Design review of the part built by this model. Coordinates are the model's own, in mm. A direction names the side the tool comes from. Give positions to 0.01 mm unless a question says otherwise; leave off trailing zeros. Write each loop counter-clockwise with the first axis right and the second up, starting at its lowest first coordinate (ties: lowest second). Pieces come first, ordered by that corner, then holes. Notation, with made-up numbers: (53.5, -13.75) -> (76.5, -13.75) arc R22 ccw to (76.5, 19.25) -> close; hole circle Ø4 at (68.25, 47). An arc over 180 degrees is marked (long way). Answer as a JSON object with one key per item and string values.
Autodesk Inventor part; units mm, degrees
ref_plane "YZ Plane" through (0, 0, 0) normal (1, 0, 0) x (0, 1, 0)
ref_plane "XZ Plane" through (0, 0, 0) normal (0, 1, 0) x (-1, 0, 0)
ref_plane "XY Plane" through (0, 0, 0) normal (0, 0, 1) x (1, 0, 0)
sketch "스케치1" plane through (0, 0, 0) normal (1, 0, 0) x (0, 1, 0)
  line L0 (0, 0) -> (15, 0)
  line L1 (15, 0) -> (15, -11)
  line L2 (15, -11) -> (0, -11)
  line L3 (0, -11) -> (0, 0)
  line L4 (15, -11) -> (8.9773, -11)
  line L5 (10, -9.9773) -> (15, -9.9773)
  line L6 (15, -9.9773) -> (15, -11)
  line L7 (0, -11) -> (5, -11)
  line L8 (0, -10) -> (0, -11)
  line L9 (5, -11) -> (7, -11)
  line L10 (7, -11) -> (8, -11)
  line L11 (8, -11) -> (8, -10.5)
  line L12 (8.9773, -11) -> (10, -9.9773)
  line L13 (8.9773, -11) -> (10.4236, -11) construction
  line L14 (7, -11) -> (7.5, -10.5)
  line L15 (8, -10.5) -> (7.5, -10.5)
  dimension "d0" = 15
  dimension "d1" = 11
  dimension "d8" = 45
  dimension "d9" = 5
extrude "돌출1" add sketch "스케치1" along normal blind 1 contours L0 L1 L5 L12 L2 L11 L15 L14 L3
fillet "모깎기1" radius 1 4 edges at (0.5, 15, -9.9773) (0.5, 15, 0) (0.5, 0, -11) (0.5, 0, 0)
sketch "스케치2" plane through (1, 0, 0) normal (1, 0, 0) x (0, 0, -1)
  arc A0 (0, 1) -> (1, 0) centre (1, 1) ccw
  line L0 (1, 0) -> (10, 0)
  arc A1 (10, 0) -> (11, 1) centre (10, 1) ccw
  line L1 (11, 1) -> (11, 7)
  line L2 (11, 7) -> (10.5, 7.5)
  line L3 (10.5, 7.5) -> (10.5, 8)
  line L4 (10.5, 8) -> (11, 8)
  line L5 (11, 8) -> (11, 8.9773)
  line L6 (11, 8.9773) -> (9.9773, 10)
  line L7 (9.9773, 10) -> (9.9773, 14)
  arc A2 (9.9773, 14) -> (8.9773, 15) centre (8.9773, 14) ccw
  line L8 (8.9773, 15) -> (1, 15)
  arc A3 (1, 15) -> (0, 14) centre (1, 14) ccw
  line L9 (0, 14) -> (0, 1)
  line L10 (-0.1139, -0.2414) -> (-0.1139, 15.1589) construction
  line L11 (-0.1139, 15.1589) -> (11.0874, 15.1589) construction
  line L12 (11.0874, 15.1589) -> (11.0874, -0.2414) construction
  line L13 (11.0874, -0.2414) -> (-0.1139, -0.2414) construction
  point P0 (0, 0)
decal "전사1"
properties part number "microsd"
(1) For line 1 along Z through (x, y) = (0.2, 13); line 2 along Y through (x, z) = (0.1, -10.25); line 3 along Y through (x, z) = (0.25, -9.5), list the stretches that pass through material, from the lowest coordinate up.
Here are the results:
{"line 1": "z = -9.98 to 0", "line 2": "y = 0.03 to 9.73", "line 3": "y = 0 to 14.85"}
(2) We need section B-B, the plane y = 13.5. State the section outline as (x, z) points, then the cut area to 3 significant figures.
Here are the results:
{"outline": "(0, -9.98) -> (1, -9.98) -> (1, 0) -> (0, 0) -> close", "area": "9.98 mm²"}
(3) For faces 1 (the flat face through (0.5, 12, -9.977)), 2 (the cylindrical face through (0.507, 0.285, -10.699)), list the 3-axis set-ups (+Z, -Z, +X, -X, +Y, -Y) from which the entire face can be reached by the end or side of a thin tool; tool diameter is ignored.
Here are the results:
{"face 1": "-Z, +X, -X, +Y", "face 2": "-Z, +X, -X, -Y"}
(4) We need section C-C, the plane z = -9.75. State the section outline as (x, y) points, then the cut area to 3 significant figures.
Here are the results:
{"outline": "(0, 0) -> (1, 0) -> (1, 14.64) -> (0, 14.64) -> close", "area": "14.6 mm²"}
(5) We need section A-A, the plane x = 0.15. State the section outline as (y, z) points.
Here are the results:
{"outline": "(0, -10) arc R1 ccw to (1, -11) -> (7, -11) -> (7.5, -10.5) -> (8, -10.5) -> (8, -11) -> (8.98, -11) -> (10, -9.98) -> (14, -9.98) arc R1 ccw to (15, -8.98) -> (15, -1) arc R1 ccw to (14, 0) -> (1, 0) arc R1 ccw to (0, -1) -> close"}
